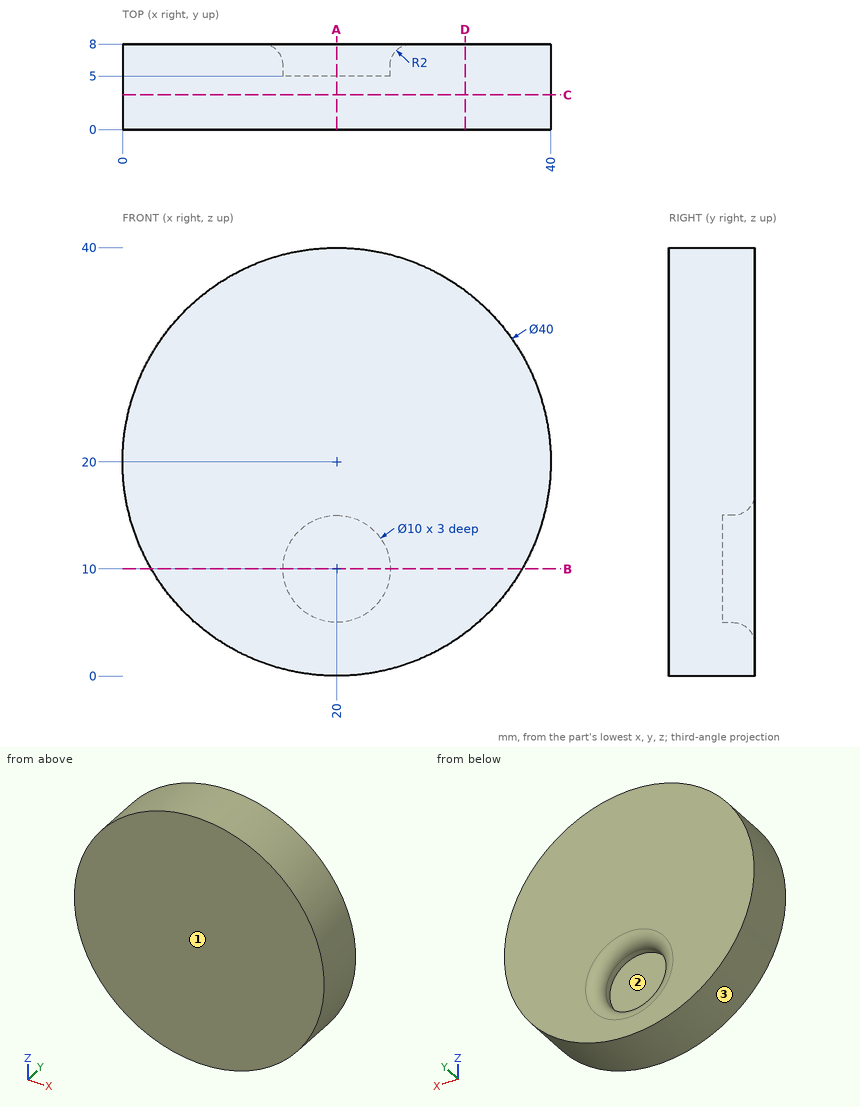
Part print with two shaded views. Sizes in mm from the minimum x, y, z corner. Round coordinates to 2 decimals unless told otherwise and drop trailing zeros. Order: outer loops, then holes, each group sorted by start corner. A loop starts at its lowest first (then second) coordinate and runs counter-clockwise, first axis right, second up.
(1) Band-saw the part on A-A (x = 20). List the corners of the cut face in (y, z), then the cut area to 3 significant figures.
(2) Band-saw the part on B-B (z = 10). List the corners of the cut face in (x, y).
(3) Drill centre lines: line 1 (X direction, y = 5.4, z = 10); line 2 (X direction, y = 5.75, z = 13) (3 decimals); line 3 (Z direction, x = 6.5, y = 2). Where is each one in solid material? Low to high.
(4) Band-saw the part on C-C (y = 3.25). List the corners of the cut face in (x, z), then the cut area to 3 significant figures.
(5) Pull direction Z, two halves, no side cores. Call the marked faces 1, 2 and 3: released by +Z, released by -Z, zero draft, split by the parting line, or undercut.
(6) Pin check, flat tips, straight feed: pin 1 (1.5 mm diameter, centred on y = 3, z = 20.5, fed in from -X); pin 2 (1.5 mm diameter, centred on y = 4.5, z = 5, fed in from +X); pin 3 (8 mm diameter, centred on x = 21, z = 8.5, fed in from +Y). Stop position of each tip, or through.
(7) Band-saw the part on D-D (x = 32). List the corners of the cut face in (y, z), then the cut area to 3 significant figures.
Verdict:
1. outline: (0, 0) - (8, 0) - (8, 3) arc R2 ccw to (6, 5) - (5, 5) - (5, 15) - (6, 15) arc R2 ccw to (8, 17) - (8, 40) - (0, 40) - close
1. area: 288 mm2
2. outline: (2.68, 0) - (37.32, 0) - (37.32, 8) - (27, 8) arc R2 ccw to (25, 6) - (25, 5) - (15, 5) - (15, 6) arc R2 ccw to (13, 8) - (2.68, 8) - close
3. line 1: x = 2.68 to 15, 25 to 37.32
3. line 2: x = 1.265 to 16, 24 to 38.735
3. line 3: z = 5.24 to 34.76
4. outline: circle Ø40 at (20, 20)
4. area: 1,260 mm2
5. face 1: zero draft
5. face 2: undercut
5. face 3: split by the parting line
6. pin 1: stops at x = 0
6. pin 2: stops at x = 34.03
6. pin 3: stops at y = 7.6
7. outline: (0, 4) - (8, 4) - (8, 36) - (0, 36) - close
7. area: 256 mm2
